Design review of the part built by this model. Coordinates are the model's own, in mm. Face numbers are marked on the shaded views. A direction names the side the tool comes from. Coordinates: 2 decimals unless noted, no trailing zeros. Loops run counter-clockwise (first coordinate to the right, second up) from the corner with the lowest first, then second, coordinate; pieces in that order, holes last. Notation, with made-up numbers: M 12,77.25 L 29,77.25 A16 ccw 29,102.25 Z; hole C -33,3.25 d9. An arc over 180 degrees is marked long. Answer as a JSON object with one key per item and string values. Group by question number.
1. Consider section B-B (y = -201.5). State the section outline as (x, z) points, then the cut area to 3 significant figures.
2. Consider section A-A (x = 72). State the section outline as (y, z) points.
3. Draft analysis for pull direction Z (two halves, no side actions). For the marked faces 1, 2, 3 and 4, state which applies: +Z half, -Z half, draft (parallel to the pull), parting line (faces both ways), or undercut.
4. Consider section C-C (x = 48). State the section outline as (y, z) points.
5. To check wall thickness, follow probe 1 along Z at (x, y) = (1.5, -248); probe 2 along Z at (x, y) = (0.8, 233); probe 3 along Y at (x, z) = (10, -16.5). State the ranges of each line that lie inside material, in increasing order.
6. Machinability: for the marked faces 5 and 6, which of the approach directions +Z, -Z, +X, -X, +Y, -Y give a long, thin tool a straight path to every point of the face, cutting with its end or side? Answer none if there is none.
7. Insertion check: pin 1 (8 mm diameter, centred on y = -133.5, z = 21.5, fed in from +X); pin 2 (5 mm diameter, centred on x = 87, y = -248, fed in from +Z). Each pin has a flat end and moves straight along its axis. Give the tip position at first contact, or say it passes through.
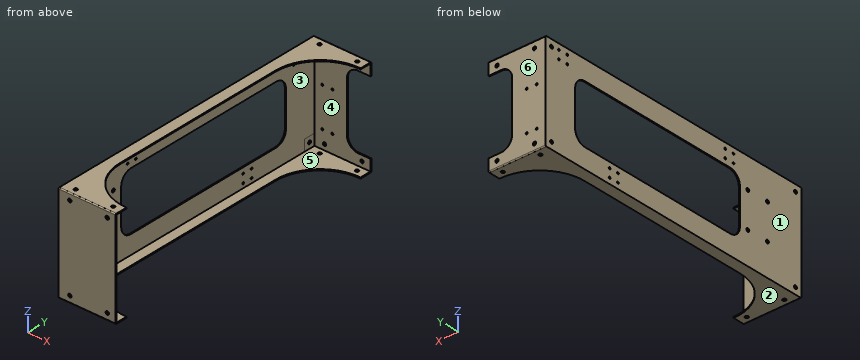
from build123d import *

# Parameters (mm, degrees)
SKETCH1_W           = 174
SKETCH1_H           = 520
BOSS_EXTRUDE1_DEPTH = 2
SKETCH2_W           = 174
SKETCH2_H           = 520
SKETCH2_W_2         = 170
SKETCH2_H_2         = 516
BOSS_EXTRUDE2_DEPTH = 100
CUT_EXTRUDE1_DEPTH  = 10
SKETCH4_R           = 3
CUT_EXTRUDE2_DEPTH  = 175
SKETCH5_R           = 3
CUT_EXTRUDE3_DEPTH  = 521
CUT_EXTRUDE4_DEPTH  = 10
SKETCH8_R           = 1.75
CUT_EXTRUDE5_DEPTH  = 10
FILLET1_R           = 1.8
SKETCH9_R           = 3
CUT_EXTRUDE6_DEPTH  = 10
SKETCH10_R          = 3
SKETCH10_R_2        = 1.75
CUT_EXTRUDE7_DEPTH  = 103
SKETCH11_W          = 20
SKETCH11_H          = 20
CUT_EXTRUDE8_DEPTH  = 0.01


with BuildPart() as part:
    # Sketch1 → Boss-Extrude1 (new body)
    with BuildSketch(Plane(origin=(0, 0, 0), x_dir=(0, 0, -1), z_dir=(1, 0, 0))):
        Rectangle(SKETCH1_W, SKETCH1_H)
    extrude(amount=BOSS_EXTRUDE1_DEPTH)

    # Sketch2 → Boss-Extrude2 (add)
    with BuildSketch(Plane(origin=(2, 0, 0), x_dir=(0, 0, -1), z_dir=(1, 0, 0))):
        Rectangle(SKETCH2_W, SKETCH2_H)
        Rectangle(SKETCH2_W_2, SKETCH2_H_2, mode=Mode.SUBTRACT)
    extrude(amount=BOSS_EXTRUDE2_DEPTH)

    # Sketch3 → Cut-Extrude1 (cut)
    with BuildSketch(Plane.XY.offset(-87)):
        with BuildLine():
            Line((102, 238), (100, 238))
            ThreePointArc((100, 238), (43.431457505, 214.568542495), (20, 158))
            Line((20, 158), (20, -158))
            ThreePointArc((20, -158), (43.431457505, -214.568542495), (100, -238))
            Line((100, -238), (102, -238))
            Line((102, -238), (102, 238))
        make_face()
    extrude(amount=CUT_EXTRUDE1_DEPTH, mode=Mode.SUBTRACT)

    # Sketch4 → Cut-Extrude2 (cut, through all)
    with BuildSketch(Plane.XY.offset(87)):
        with Locations((20, 248)):
            Circle(SKETCH4_R)
        with Locations((87, 248)):
            Circle(SKETCH4_R)
        with Locations((20, -248)):
            Circle(SKETCH4_R)
        with Locations((87, -248)):
            Circle(SKETCH4_R)
    extrude(amount=-CUT_EXTRUDE2_DEPTH, mode=Mode.SUBTRACT)

    # Sketch5 → Cut-Extrude3 (cut, through all)
    with BuildSketch(Plane(origin=(0, 260, 0), x_dir=(1, 0, 0), z_dir=(0, 1, 0))):
        with Locations(Location((87, 75, 0), (0, 0, 270))):  # turned: the seam where the file's is
            Circle(SKETCH5_R)
        with Locations(Location((20, 75, 0), (0, 0, 270))):  # turned: the seam where the file's is
            Circle(SKETCH5_R)
        with Locations(Location((87, -75, 0), (0, 0, 270))):  # turned: the seam where the file's is
            Circle(SKETCH5_R)
        with Locations(Location((20, -75, 0), (0, 0, 270))):  # turned: the seam where the file's is
            Circle(SKETCH5_R)
    extrude(amount=-CUT_EXTRUDE3_DEPTH, mode=Mode.SUBTRACT)

    # Sketch7 → Cut-Extrude4 (cut)
    with BuildSketch(Plane(origin=(0, 0, 87), x_dir=(-1, 0, 0), z_dir=(0, 0, -1))):
        with BuildLine():
            Line((-102, 238), (-100, 238))
            ThreePointArc((-100, 238), (-43.431457505, 214.568542495), (-20, 158))
            Line((-20, 158), (-20, -158))
            ThreePointArc((-20, -158), (-43.431457505, -214.568542495), (-100, -238))
            Line((-100, -238), (-102, -238))
            Line((-102, -238), (-102, 238))
        make_face()
    extrude(amount=CUT_EXTRUDE4_DEPTH, mode=Mode.SUBTRACT)

    # Sketch8 → Cut-Extrude5 (cut)
    with BuildSketch(Plane(origin=(0, 260, 0), x_dir=(1, 0, 0), z_dir=(0, 1, 0))):
        with Locations(Location((34, 53.15, 0), (0, 0, 270))):  # turned: the seam where the file's is
            Circle(SKETCH8_R)
        with Locations(Location((16, 53.15, 0), (0, 0, 270))):  # turned: the seam where the file's is
            Circle(SKETCH8_R)
        with Locations(Location((16, -16.85, 0), (0, 0, 270))):  # turned: the seam where the file's is
            Circle(SKETCH8_R)
        with Locations(Location((34, -16.85, 0), (0, 0, 270))):  # turned: the seam where the file's is
            Circle(SKETCH8_R)
        with BuildLine():
            Line((102, 65), (80, 65))
            ThreePointArc((80, 65), (65.857864376, 59.142135624), (60, 45))
            Line((60, 45), (60, -45))
            ThreePointArc((60, -45), (65.857864376, -59.142135624), (80, -65))
            Line((80, -65), (102, -65))
            Line((102, -65), (102, 65))
        make_face()
    extrude(amount=-CUT_EXTRUDE5_DEPTH, mode=Mode.SUBTRACT)

    # Fillet1
    fillet1_edges = [part.edges().sort_by_distance(p)[0] for p in [
        (51, 260, 87),
        (51, 260, -87),
        (51, -260, -87),
        (51, -260, 87),
    ]]
    fillet(fillet1_edges, radius=FILLET1_R)

    # Sketch9 → Cut-Extrude6 (cut)
    with BuildSketch(Plane.ZY):
        with Locations((-75, 248)):
            Circle(SKETCH9_R)
        with Locations((75, 248)):
            Circle(SKETCH9_R)
        with Locations((75, -248)):
            Circle(SKETCH9_R)
        with Locations((-75, -248)):
            Circle(SKETCH9_R)
    extrude(amount=-CUT_EXTRUDE6_DEPTH, mode=Mode.SUBTRACT)

    # Sketch10 → Cut-Extrude7 (cut, through all)
    with BuildSketch(Plane.ZY):
        with Locations((-29.65, -151)):
            Circle(SKETCH10_R)
        with Locations((33.35, -151)):
            Circle(SKETCH10_R)
        with Locations((-29.65, -191)):
            Circle(SKETCH10_R)
        with Locations((33.35, -191)):
            Circle(SKETCH10_R)
        with Locations((62, 233)):
            Circle(SKETCH10_R_2)
        with Locations((77, 233)):
            Circle(SKETCH10_R_2)
        with Locations((62, 216)):
            Circle(SKETCH10_R_2)
        with Locations((77, 216)):
            Circle(SKETCH10_R_2)
        with Locations((-77, 130)):
            Circle(SKETCH10_R_2)
        with Locations((-62, 130)):
            Circle(SKETCH10_R_2)
        with Locations((-62, 113)):
            Circle(SKETCH10_R_2)
        with Locations((-77, 113)):
            Circle(SKETCH10_R_2)
        with Locations((62, -105)):
            Circle(SKETCH10_R_2)
        with Locations((77, -105)):
            Circle(SKETCH10_R_2)
        with Locations((62, -122)):
            Circle(SKETCH10_R_2)
        with Locations((77, -122)):
            Circle(SKETCH10_R_2)
        with BuildLine():
            Line((-32, 200), (32, 200))
            ThreePointArc((32, 200), (46.142135624, 194.142135624), (52, 180))
            Line((52, 180), (52, -115))
            ThreePointArc((52, -115), (46.142135624, -129.142135624), (32, -135))
            Line((32, -135), (-32, -135))
            ThreePointArc((-32, -135), (-46.142135624, -129.142135624), (-52, -115))
            Line((-52, -115), (-52, 180))
            ThreePointArc((-52, 180), (-46.142135624, 194.142135624), (-32, 200))
        make_face()
    extrude(amount=-CUT_EXTRUDE7_DEPTH, mode=Mode.SUBTRACT)

    # Sketch11 → Cut-Extrude8 (cut)
    with BuildSketch(Plane(origin=(2, 0, 0), x_dir=(0, 0, -1), z_dir=(1, 0, 0))):
        with Locations((-75, 248)):
            Rectangle(SKETCH11_W, SKETCH11_H)
        with Locations((75, 248)):
            Rectangle(SKETCH11_W, SKETCH11_H)
        with Locations((75, -248)):
            Rectangle(SKETCH11_W, SKETCH11_H)
        with Locations((-75, -248)):
            Rectangle(SKETCH11_W, SKETCH11_H)
    extrude(amount=-CUT_EXTRUDE8_DEPTH, mode=Mode.SUBTRACT)


solid = part.part
Findings below:
{
 "1": {"outline": "M 0,-87 L 32.86,-87 L 32.86,-85 L 2,-85 L 2,85 L 32.86,85 L 32.86,87 L 0,87 Z", "area": "471 mm^2"},
 "2": {"outline": "M -260,-85.2 A1.8 ccw -258.2,-87 L -232.94,-87 L -232.94,-85 L -258,-85 L -258,85 L -232.94,85 L -232.94,87 L -258.2,87 A1.8 ccw -260,85.2 Z; M 232.94,-87 L 258.2,-87 A1.8 ccw 260,-85.2 L 260,-63.33 L 258,-63.33 L 258,-85 L 232.94,-85 Z; M 232.94,85 L 258,85 L 258,63.33 L 260,63.33 L 260,85.2 A1.8 ccw 258.2,87 L 232.94,87 Z"},
 "3": {"face 1": "draft", "face 2": "-Z half", "face 3": "undercut", "face 4": "undercut"},
 "4": {"outline": "M -260,-85.2 A1.8 ccw -258.2,-87 L -218.79,-87 L -218.79,-85 L -258,-85 L -258,85 L -218.79,85 L -218.79,87 L -258.2,87 A1.8 ccw -260,85.2 Z; M 218.79,-87 L 258.2,-87 A1.8 ccw 260,-85.2 L 260,85.2 A1.8 ccw 258.2,87 L 218.79,87 L 218.79,85 L 258,85 L 258,-85 L 218.79,-85 Z"},
 "5": {"probe 1": "z = -87 to -78, -72 to 72, 78 to 87", "probe 2": "z = -87 to 60.25, 63.75 to 75.25, 78.75 to 87", "probe 3": "y = -260 to -258, 258 to 260"},
 "6": {"face 5": "+X", "face 6": "+Z, -Z, +X, -X, +Y"},
 "7": {"pin 1": "stops at x = 2", "pin 2": "passes through"}
}
